The model under review builds one solid part; all positions refer to its coordinate system, in mm. A direction names the side the tool comes from. Round coordinates to 2 decimals unless told otherwise and drop trailing zeros. Loops run counter-clockwise (first coordinate to the right, second up) from the corner with the lowest first, then second, coordinate; pieces in that order, holes last. Notation, with made-up numbers: M 59,-19.5 L 82,-19.5 A25 cw 82,15.5 Z; hole C 87.5,39 d6. An arc over 180 degrees is marked long. One line per question, with ' | ' between items.
from build123d import *

# Parameters (mm, degrees)
BOSS_EXTRUDE1_DEPTH = 10
SKETCH2_R           = 3.5
CUT_EXTRUDE1_DEPTH  = 10
SKETCH3_R           = 6
CUT_EXTRUDE2_DEPTH  = 48.707441768
FILLET1_R           = 2


with BuildPart() as part:
    # Sketch1 → Boss-Extrude1 (new body)
    with BuildSketch(Plane(origin=(0, 0, 0), x_dir=(1, 0, 0), z_dir=(0, 1, 0))):
        Polygon((-10, -10), (-20, -10), (-20, 10), (20, 10), (20, -10), (10, -10), (10, -24), (-10, -24), align=None)
    extrude(amount=BOSS_EXTRUDE1_DEPTH)

    # Sketch2 → Cut-Extrude1 (cut)
    with BuildSketch(Plane(origin=(0, 10, 0), x_dir=(1, 0, 0), z_dir=(0, 1, 0))):
        with Locations(Location((0, -17, 0), (0, 0, 270))):
            Circle(SKETCH2_R)
    extrude(amount=-CUT_EXTRUDE1_DEPTH, mode=Mode.SUBTRACT)

    # Sketch3 → Cut-Extrude2 (cut, through all)
    with BuildSketch(Plane(origin=(20, 0, 0), x_dir=(0, 0, -1), z_dir=(1, 0, 0))):
        with Locations((0, 10)):
            Circle(SKETCH3_R)
    extrude(amount=-CUT_EXTRUDE2_DEPTH, mode=Mode.SUBTRACT)

    # Fillet1
    fillet1_edges = [part.edges().sort_by_distance(p)[0] for p in [
        (-20, 5, -10),
        (20, 5, -10),
        (20, 5, 10),
        (10, 5, 10),
        (10, 5, 24),
        (-10, 5, 24),
        (-10, 5, 10),
        (-20, 5, 10),
    ]]
    fillet(fillet1_edges, radius=FILLET1_R)


solid = part.part
1) Add section D-D on x = -14. State the section outline as (y, z) points.
Output values:
outline: M 0,-10 L 10,-10 L 10,-6 A6 cw 10,6 L 10,10 L 0,10 Z
2) Mouldability with a two-part tool opening along Z and no side actions: class faces 1 (the cylindrical face through (0, 4, 0)), 2 (the flat face through (0, 5, -10)), 3 (the flat face through (0, 10, -8)) as +Z half, -Z half, draft (parallel to the pull), parting line (faces both ways), or undercut.
Output values:
face 1: undercut | face 2: -Z half | face 3: draft
3) For line 1 (X direction, y = 7, z = 17); line 2 (Z direction, x = 0.5, y = 7); line 3 (Z direction, x = -12, y = 9.75), list the stretches that pass through material, from the lowest coordinate up.
Output values:
line 1: x = -10 to -3.5, 3.5 to 10 | line 2: z = -10 to -5.2, 5.2 to 13.54, 20.46 to 24 | line 3: z = -10 to -5.99, 5.99 to 10
4) Add section C-C on x = 0.5. State the section outline as (y, z) points, then the cut area to 3 significant figures.
Output values:
outline: M 0,-10 L 10,-10 L 10,-6 A6 cw 10,6 L 10,13.54 L 0,13.54 Z; M 0,20.46 L 10,20.46 L 10,24 L 0,24 Z | area: 214 mm²
5) Add section B-B on z = 17. State the section outline as (x, y) points.
Output values:
outline: M -10,0 L -3.5,0 L -3.5,10 L -10,10 Z; M 3.5,0 L 10,0 L 10,10 L 3.5,10 Z
6) Insertion check: P1, Ø4, axis at y = 5.5, z = 11.5, coming from the -X side; P2, Ø5, axis at y = 3, z = 16.5, coming from the +X side; P3, Ø6.5, axis at x = 0, z = 17, coming from the -Y side; P4, Ø1.8, axis at x = -15, y = 7, coming from the +Z side. Each pin has a flat end and moves straight along its axis. Give the tip position at first contact, or say it passes through.
Output values:
P1: stops at x = -19.32 | P2: stops at x = 10 | P3: passes through | P4: stops at z = 10
7) Machinability: for faces 4 (the flat face through (10, 5, 17)), 5 (the cylindrical face through (-19.43, 5.07, -9.4)), 6 (the flat face through (-10, 5, 17)), which of the approach directions +Z, -Z, +X, -X, +Y, -Y give a long, thin tool a straight path to every point of the face, cutting with its end or side? Answer none if there is none.
Output values:
face 4: +Z, +X, +Y, -Y | face 5: -Z, -X, +Y, -Y | face 6: +Z, -X, +Y, -Y
8) Add section A-A on y = 5. State the section outline as (x, z) points, then the cut area to 3 significant figures.
Output values:
outline: M -20,-8 A2 ccw -18,-10 L 18,-10 A2 ccw 20,-8 L 20,-3.32 L -20,-3.32 Z; M -20,3.32 L 20,3.32 L 20,8 A2 ccw 18,10 L 12,10 A2 cw 10,12 L 10,22 A2 ccw 8,24 L -8,24 A2 ccw -10,22 L -10,12 A2 cw -12,10 L -18,10 A2 ccw -20,8 Z; hole C 0,17 d7 | area: 773 mm²
